Verification items for the finished model (mm, model axes). Face numbers are marked on the shaded views. A direction names the side the tool comes from. Give positions to 0.01 mm unless a question says otherwise; leave off trailing zeros. Write each loop counter-clockwise with the first axis right and the second up, starting at its lowest first coordinate (ties: lowest second). Pieces come first, ordered by that corner, then holes. Notation, with made-up numbers: (31.5, 27.25) -> (67.5, 27.25) arc R22 ccw to (67.5, 64.25) -> close; hole circle Ø7 at (50, 62). An arc over 180 degrees is marked (long way). Answer as CSV lines item,"result".
```python
from build123d import *

# Parameters (mm, degrees)
SKETCH_1_W      = 10.16
SKETCH_1_H      = 10.16
EXTRUDE_1_DEPTH = 3


with BuildPart() as part:
    # 스케치1 → 보스-돌출1 (new body)
    with BuildSketch(Plane(origin=(0, 0, 0), x_dir=(1, 0, 0), z_dir=(0, 1, 0))):
        with BuildLine():
            Line((6.88975, 6.0198), (6.88975, 7.4958))
            ThreePointArc((6.88975, 7.4958), (6.443380735, 8.573430735), (5.36575, 9.0198))
            Line((5.36575, 9.0198), (5.08, 9.0198))
            Line((5.08, 9.0198), (-5.08, 9.0198))
            Line((-5.08, 9.0198), (-6.88975, 9.0198))
            Line((-6.88975, 9.0198), (-6.88975, 5.8702))
            Line((-6.88975, 5.8702), (-9.88975, 5.8702))
            Line((-9.88975, 5.8702), (-9.88975, -3.0198))
            Line((-9.88975, -3.0198), (-6.88975, -3.0198))
            Line((-6.88975, -3.0198), (-6.88975, -6.0198))
            Line((-6.88975, -6.0198), (-3.81, -6.0198))
            Line((-3.81, -6.0198), (-3.81, -9.0198))
            Line((-3.81, -9.0198), (3.81, -9.0198))
            Line((3.81, -9.0198), (3.81, -6.0198))
            Line((3.81, -6.0198), (6.88975, -6.0198))
            Line((6.88975, -6.0198), (6.88975, 6.0198))
        make_face()
        with Locations((0, 0.9398)):
            Rectangle(SKETCH_1_W, SKETCH_1_H, mode=Mode.SUBTRACT)
    extrude(amount=-EXTRUDE_1_DEPTH)


solid = part.part
```
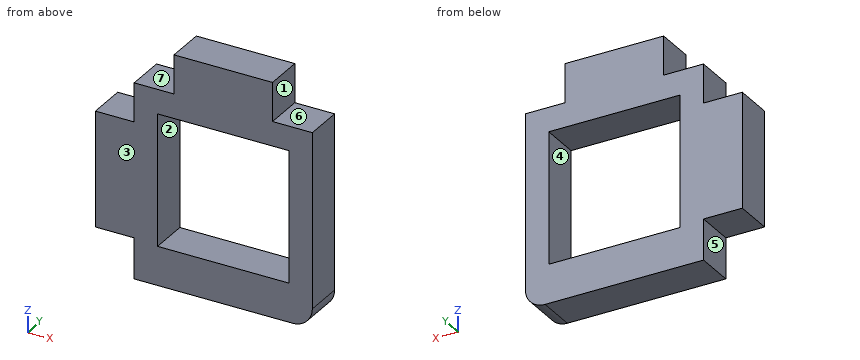
1) Section check B-B (x = 0). Record the boundary of the cut face in (y, z), and give its area (3 significant figures).
Reported:
outline,"(-3, -9.02) -> (0, -9.02) -> (0, -6.02) -> (-3, -6.02) -> close; (-3, 4.14) -> (0, 4.14) -> (0, 9.02) -> (-3, 9.02) -> close"
area,"23.6 mm²"
2) Scan lines: line 1 along Z through (x, y) = (-1.5, -2.15); line 2 along X through (y, z) = (-2.75, 2); line 3 along Z through (x, y) = (5, -2.7). Record each from-to range of solid material in increasing order.
Reported:
line 1,"-9.02 to -6.02, 4.14 to 9.02"
line 2,"-9.89 to -5.08, 5.08 to 6.89"
line 3,"-9.02 to -6.02, 4.14 to 6.02"
3) Section check A-A (z = 2.25). Record the boundary of the cut face in (x, y), and give its area (3 significant figures).
Reported:
outline,"(-9.89, -3) -> (-5.08, -3) -> (-5.08, 0) -> (-9.89, 0) -> close; (5.08, -3) -> (6.89, -3) -> (6.89, 0) -> (5.08, 0) -> close"
area,"19.9 mm²"
4) Section check C-C (y = -2.2). Record the boundary of the cut face in (x, z).
Reported:
outline,"(-9.89, -5.87) -> (-6.89, -5.87) -> (-6.89, -9.02) -> (5.37, -9.02) arc R1.52 ccw to (6.89, -7.5) -> (6.89, 6.02) -> (3.81, 6.02) -> (3.81, 9.02) -> (-3.81, 9.02) -> (-3.81, 6.02) -> (-6.89, 6.02) -> (-6.89, 3.02) -> (-9.89, 3.02) -> close; hole (-5.08, -6.02) -> (5.08, -6.02) -> (5.08, 4.14) -> (-5.08, 4.14) -> close"
5) Section check D-D (x = -6). Record the boundary of the cut face in (y, z), and give its area (3 significant figures).
Reported:
outline,"(-3, -9.02) -> (0, -9.02) -> (0, 6.02) -> (-3, 6.02) -> close"
area,"45.1 mm²"
6) Draft check along X on the marked faces 1, 2 and 3. Enter one of: +X half, -X half, draft (parallel to the pull), parting line (faces both ways), or undercut.
Reported:
face 1,"+X half"
face 2,"undercut"
face 3,"draft"
7) Tool access check on the marked faces 4, 5, 6 and 7. Record the directions out of +Z, -Z, +X, -X, +Y, -Y that give a thin tool (end or side, any length) a straight path to the whole face; none if there is none.
Reported:
face 4,"+Y, -Y"
face 5,"-Z, -X, +Y, -Y"
face 6,"+Z, +X, +Y, -Y"
face 7,"+Z, -X, +Y, -Y"
8) Depth check by flat-ended pin: pin 1 (1.5 mm diameter, centred on y = -1, z = 4.5, fed in from -X); pin 2 (1.5 mm diameter, centred on x = -9, y = -1, fed in from -Z); pin 3 (2 mm diameter, centred on x = -7.5, z = -6.5, fed in from +Y); pin 4 (0.9 mm diameter, centred on x = -6, y = -2, fed in from +Z). Enter the tip coordinate at first touch or a pass-through.
Reported:
pin 1,"x = -6.89"
pin 2,"z = -5.87"
pin 3,"y = 0"
pin 4,"z = 6.02"
